Verification items for the finished model (mm, model axes). Coordinates: 2 decimals unless noted, no trailing zeros. Write each loop counter-clockwise with the first axis right and the second up, starting at its lowest first coordinate (ties: lowest second). Pieces come first, ordered by that corner, then holes. Notation, with made-up numbers: (-37, 32.5) -> (-20, 32.5) arc R18 cw to (-20, 51.5) -> close; hole circle Ø5 at (22.5, 58). An arc over 180 degrees is marked (long way). Answer in a Markdown table with one row per item.
```python
from build123d import *

# Parameters (mm, degrees)
SKETCH1_W           = 36.5125
SKETCH1_H           = 79.375
BOSS_EXTRUDE1_DEPTH = 7.9375
SKETCH2_W           = 36.5125
SKETCH2_H           = 79.375
SKETCH2_W_2         = 23.8125
SKETCH2_H_2         = 69.215
CUT_EXTRUDE1_DEPTH  = 2.54


with BuildPart() as part:
    # Sketch1 → Boss-Extrude1 (new body)
    with BuildSketch(Plane(origin=(0, 0, 0), x_dir=(1, 0, 0), z_dir=(0, 1, 0))):
        with Locations((18.25625, 39.6875)):
            Rectangle(SKETCH1_W, SKETCH1_H)
    extrude(amount=BOSS_EXTRUDE1_DEPTH)

    # Sketch2 → Cut-Extrude1 (cut)
    with BuildSketch(Plane(origin=(0, 7.9375, 0), x_dir=(1, 0, 0), z_dir=(0, 1, 0))):
        with Locations((18.25625, 39.6875)):
            Rectangle(SKETCH2_W, SKETCH2_H)
        with Locations((18.25625, 39.6875)):
            Rectangle(SKETCH2_W_2, SKETCH2_H_2, mode=Mode.SUBTRACT)
    extrude(amount=-CUT_EXTRUDE1_DEPTH, mode=Mode.SUBTRACT)


solid = part.part
```
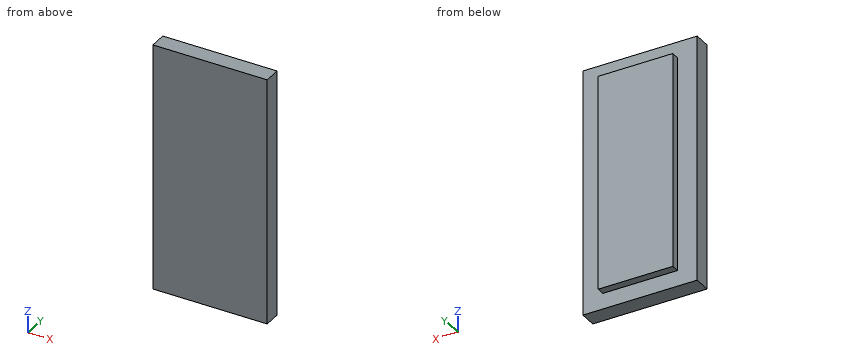
1. Section check B-B, the plane z = -32. Record the boundary of the cut face in (x, y), plus the area to 3 significant figures.
Geometry says:
| item | result |
|---|---|
| outline | (0, 0) -> (36.51, 0) -> (36.51, 5.4) -> (30.16, 5.4) -> (30.16, 7.94) -> (6.35, 7.94) -> (6.35, 5.4) -> (0, 5.4) -> close |
| area | 258 mm^2 |
2. Section check D-D, the plane x = 5. Record the boundary of the cut face in (y, z) (1 decimal).
Geometry says:
| item | result |
|---|---|
| outline | (0, -79.4) -> (5.4, -79.4) -> (5.4, 0) -> (0, 0) -> close |
3. Thickness scan on line 1 (X direction, y = 7.25, z = -42); line 2 (Y direction, x = 4.5, z = -57.5); line 3 (Z direction, x = 27, y = 7) (3 decimals). Record the ranges inside material, lowest first. Write a range as from..to.
Geometry says:
| item | result |
|---|---|
| line 1 | 6.35..30.16 |
| line 2 | 0..5.4 |
| line 3 | -74.295..-5.08 |
4. Depth check by flat-ended pin: P1, Ø1.3, axis at y = 7, z = -32, coming from the -X side; P2, Ø2, axis at y = 6.5, z = -44.5, coming from the +X side; P3, Ø0.8, axis at x = 24, y = 6, coming from the -Z side (3 decimals). Enter the tip coordinate at first touch or a pass-through.
Geometry says:
| item | result |
|---|---|
| P1 | x = 6.35 |
| P2 | x = 30.16 |
| P3 | z = -74.295 |
5. Section check A-A, the plane x = 22. Record the boundary of the cut face in (y, z) (1 decimal), plus the area to 3 significant figures.
Geometry says:
| item | result |
|---|---|
| outline | (0, -79.4) -> (5.4, -79.4) -> (5.4, -74.3) -> (7.9, -74.3) -> (7.9, -5.1) -> (5.4, -5.1) -> (5.4, 0) -> (0, 0) -> close |
| area | 604 mm^2 |
